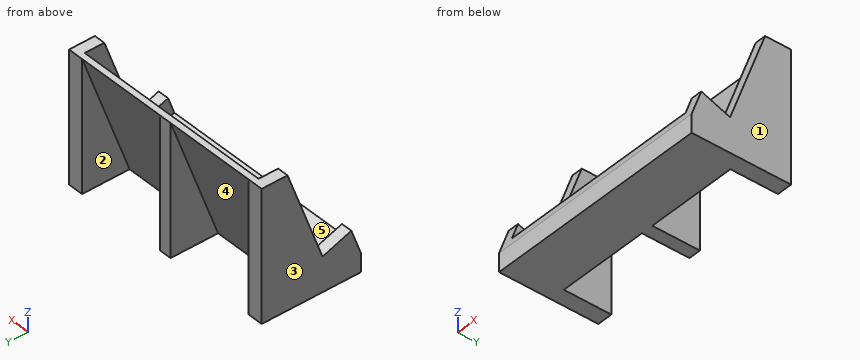
from build123d import *

# Parameters (mm, degrees)
F0_W      = 40
F0_H      = 112.7631144943
F1_DEPTH  = 92.5
F2_W      = 167
F2_H      = 104
F3_DEPTH  = 40
F4_W      = 19.1075097164
F4_H      = 21.1983466993
F5_DEPTH  = 200
F7_DEPTH  = 200
F9_DEPTH  = 80
F10_DEPTH = 5


with BuildPart() as f1:
    # F0 (on Right) → F1 (new body, symmetric)
    with BuildSketch(Plane.YZ):
        Polygon((41.0424171991, 112.7631144943), (0, 0), (41.0424171991, 0), align=None)
        Polygon((41.0424171991, 0), (0, 0), (0, -15), (81.0424171991, -15), (81.0424171991, 0), align=None)
        with Locations((61.0424171991, 56.3815572472)):
            Rectangle(F0_W, F0_H)
    extrude(amount=F1_DEPTH, both=True)

    # F2 (on face) → F3 (cut)
    with BuildSketch(Plane(origin=(0, 0, 0), x_dir=(1, 0, 0), z_dir=(0, -0.9396926208, 0.3420201433))):
        with Locations((0, 60)):
            Rectangle(F2_W, F2_H)
    extrude(amount=-F3_DEPTH, mode=Mode.SUBTRACT)

    # F4 (on face) → F5 (cut)
    with BuildSketch(Plane.YZ.offset(92.5)):
        with Locations((90.5961720573, 102.1639411447)):
            Rectangle(F4_W, F4_H)
        Polygon((81.0424171991, 91.564767795), (81.0424171991, 112.7631144943), (41.0424171991, 112.7631144943), (33.3268499849, 91.564767795), align=None)
        Polygon((33.3268499849, 91.564767795), (41.0424171991, 112.7631144943), (33.0099269154, 112.7631144943), (33.0099269154, 91.564767795), align=None)
    extrude(amount=-F5_DEPTH, mode=Mode.SUBTRACT)

    # F6 (on face) → F7 (cut)
    with BuildSketch(Plane.YZ.offset(92.5)):
        Polygon((33.3268499849, 91.564767795), (7.8664632965, 21.6129302781), (31.3587788161, 13.0624266949), (59.9312942968, 91.564767795), align=None)
    extrude(amount=-F7_DEPTH, mode=Mode.SUBTRACT)

    # F8 (on Right) → F9 (cut, symmetric)
    with BuildSketch(Plane.YZ):
        Polygon((81.0424171991, -15), (81.0424171991, 91.564767795), (42.2560137002, -15), align=None)
    extrude(amount=F9_DEPTH, both=True, mode=Mode.SUBTRACT)

    # F8 (on Right) → F10 (join, symmetric)
    with BuildSketch(Plane.YZ):
        Polygon((81.0424171991, -15), (81.0424171991, 91.564767795), (42.2560137002, -15), align=None)
    extrude(amount=F10_DEPTH, both=True)


solid = f1.part
Read the model definition and answer for the solid it produces. Units are mm, in the model's axes. Face numbers are marked on the shaded views. A direction names the side the tool comes from. Coordinates: 2 decimals unless noted, no trailing zeros. Loops run counter-clockwise (first coordinate to the right, second up) from the corner with the lowest first, then second, coordinate; pieces in that order, holes last.
Q1. The part is cut by section D-D on y = 16.5. Write down the section's boundary in (x, z), and give its area (3 significant figures).
Q2. The part is cut by section A-A on x = -71. Write down the section's boundary in (y, z).
Q3. Each of these flat-tipped pins is pushed along its axis until it touches: pin 1 Ø4 at (x, z) = (-60.5, 54.5) entering from +Y; pin 2 Ø6 at (x, z) = (70, 18.5) entering from -Y; pin 3 Ø12 at (x, z) = (-45, 5.5) entering from +Y. Where does it stop, or does it pass through?
Q4. Which of the six approach directions +Z, -Z, +X, -X, +Y, -Y give full straight-line access (tool end or side, diameter ignored) to the marked faces 1 and 2?
Q5. Consider probe 1 along X at (y, z) = (56.5, -1); probe 2 along X at (y, z) = (9, 10.5); probe 3 along Z at (x, y) = (-18, 23.5). Determine where each line is inside the solid, lowest interval first.
Q6. The part is cut by section B-B on z = -4. Write down the section's boundary in (x, y), and give its area (3 significant figures).
Q7. The part is cut by section C-C on z = 15. Write down the section's boundary in (x, y).
Q8. The mould has two halves that part along Y. Classify the marked faces 3, 4 and 5: +Y half, -Y half, draft (parallel to the pull), parting line (faces both ways), or undercut.
Results below:
1. outline: (-92.5, -15) - (92.5, -15) - (92.5, 18.47) - (83.5, 18.47) - (83.5, 2.51) - (-83.5, 2.51) - (-83.5, 18.47) - (-92.5, 18.47) - close
1. area: 3,530 mm2
2. outline: (0, -15) - (42.26, -15) - (81.04, 91.56) - (75.89, 91.56) - (40.32, -6.16) - (2.74, 7.52) - (0, 0) - close
3. pin 1: stops at y = 68.28
3. pin 2: stops at y = 48.21
3. pin 3: stops at y = 51.9
4. face 1: +Z, -Z, +X, +Y, -Y
4. face 2: -Z, +Y
5. probe 1: x = -92.5 to -80, -5 to 5, 80 to 92.5
5. probe 2: x = -92.5 to -83.5, 83.5 to 92.5
5. probe 3: z = -15 to -0.04
6. outline: (-92.5, 0) - (92.5, 0) - (92.5, 81.04) - (80, 81.04) - (80, 46.26) - (5, 46.26) - (5, 81.04) - (-5, 81.04) - (-5, 46.26) - (-80, 46.26) - (-80, 81.04) - (-92.5, 81.04) - close; hole (-83.5, 34.38) - (83.5, 34.38) - (83.5, 41.11) - (-83.5, 41.11) - close
6. area: 8,650 mm2
7. outline: (-92.5, 5.46) - (-83.5, 5.46) - (-83.5, 26.04) - (-92.5, 26.04) - close; (-92.5, 32.06) - (-83.5, 32.06) - (-83.5, 48.03) - (83.5, 48.03) - (83.5, 32.06) - (92.5, 32.06) - (92.5, 81.04) - (80, 81.04) - (80, 53.18) - (5, 53.18) - (5, 81.04) - (-5, 81.04) - (-5, 53.18) - (-80, 53.18) - (-80, 81.04) - (-92.5, 81.04) - close; (83.5, 5.46) - (92.5, 5.46) - (92.5, 26.04) - (83.5, 26.04) - close
8. face 3: draft
8. face 4: +Y half
8. face 5: undercut
